Autodesk Inventor part; units mm, degrees
ref_plane "YZ Plane" through (0, 0, 0) normal (1, 0, 0) x (0, 1, 0)
ref_plane "XZ Plane" through (0, 0, 0) normal (0, 1, 0) x (-1, 0, 0)
ref_plane "XY Plane" through (0, 0, 0) normal (0, 0, 1) x (1, 0, 0)
ref_plane "Work Plane1" through (0, 0, 0) normal (0, 0, 1) x (1, 0, 0)
sketch "Sketch1" plane through (0, 0, 0) normal (0, 0, 1) x (1, 0, 0)
  circle A0 centre (6.5, 20.75) radius 1
  circle A1 centre (6.5, 4.75) radius 1
  circle A2 centre (22.5, 20.75) radius 1
  circle A3 centre (22.5, 4.75) radius 1
  line L0 (-13, -14.75) -> (43.896, -14.75)
  line L1 (43.896, -14.75) -> (43.896, 40.25)
  line L2 (43.896, 40.25) -> (-13, 40.25)
  line L3 (-13, 40.25) -> (-13, -14.75)
  circle A4 centre (22.5, 12.75) radius 1
  circle A5 centre (14.5, 20.75) radius 1
  circle A6 centre (14.5, 4.75) radius 1
  circle A7 centre (6.5, 12.75) radius 1
  point P0 (0, 0)
  point P1 (14.5, 12.75)
  dimension "d1" = 55
  dimension "d102" = 29.396
  dimension "d103" = 27.5
  dimension "d107" = 2
  dimension "d108" = 2
  dimension "d109" = 2
  dimension "d110" = 2
extrude "Extrusion3" add sketch "Sketch1" along normal blind 3
sketch "Sketch4" plane through (0, 0, 3) normal (0, 0, 1) x (1, 0, 0)
  line L0 (42, 40.25) -> (-13, 40.25) construction
  line L1 (14.5, 40.25) -> (14.5, 12.75) construction
  line L2 (-13, -14.75) -> (42, -14.75) construction
  line L3 (-13, 40.25) -> (-13, -14.75) construction
  line L4 (-13, 12.75) -> (14.5, 12.75) construction
  circle A0 centre (14.5, 30.75) radius 3.895
  circle A1 centre (1.7721, 25.4779) radius 3.895
  circle A2 centre (-3.5, 12.75) radius 3.895
  circle A3 centre (1.7721, 0.0221) radius 3.895
  circle A4 centre (14.5, -5.25) radius 3.895
  circle A5 centre (27.2279, 0.0221) radius 3.895
  circle A6 centre (32.5, 12.75) radius 3.895
  circle A7 centre (27.2279, 25.4779) radius 3.895
  arc A8 (4.6716, 35.75) -> (4.6716, 37.75) centre (7.5, 36.75) ccw
  line L5 (42, 40.25) -> (-13, 40.25)
  line L6 (7.5, 36.75) -> (-13, 36.75) construction
  line L7 (4.6716, 37.75) -> (-7.3284, 37.75)
  line L8 (4.6716, 35.75) -> (-7.3284, 35.75)
  line L9 (-7.3284, 37.75) -> (-7.3284, 40.25)
  line L10 (10.9716, 40.25) -> (-7.3284, 40.25)
  line L11 (-7.3284, 35.75) -> (-7.3284, 33.25)
  line L12 (-7.3284, 33.25) -> (10.9716, 33.25)
  line L13 (10.9716, 40.25) -> (10.9716, 33.25)
  arc A9 (24.3284, 37.75) -> (24.3284, 35.75) centre (21.5, 36.75) ccw
  line L14 (24.3284, 37.75) -> (36.3284, 37.75)
  line L15 (24.3284, 35.75) -> (36.3284, 35.75)
  line L16 (36.3284, 37.75) -> (36.3284, 40.25)
  line L17 (18.0284, 40.25) -> (36.3284, 40.25)
  line L18 (36.3284, 35.75) -> (36.3284, 33.25)
  line L19 (36.3284, 33.25) -> (18.0284, 33.25)
  line L20 (18.0284, 40.25) -> (18.0284, 33.25)
  arc A10 (-6.6716, -10.25) -> (-6.6716, -12.25) centre (-9.5, -11.25) ccw
  line L21 (-9.5, -11.25) -> (8.4531, -11.25) construction
  line L22 (-6.6716, -10.25) -> (5.3284, -10.25)
  line L23 (-6.6716, -12.25) -> (5.3284, -12.25)
  line L24 (5.3284, -12.25) -> (5.3284, -14.75)
  line L25 (5.3284, -10.25) -> (5.3284, -7.75)
  line L26 (5.3284, -7.75) -> (-13, -7.75)
  line L27 (-13, -14.75) -> (-13, -7.75)
  line L28 (-13, -14.75) -> (5.3284, -14.75)
  circle A11 centre (14.5, 12.75) radius 5
  point P0 (0, 0)
  dimension "d24" = 7.79
  dimension "d25" = 18
  dimension "d28" = 360
  dimension "d63" = 6
  dimension "d64" = 7
  dimension "d65" = 12
  dimension "d66" = 18.3
  dimension "d67" = 2.5
  dimension "d68" = 3.5
  dimension "d71" = 1
  dimension "d74" = 6
  dimension "d75" = 3.5
  dimension "d76" = 3.5
  dimension "d77" = 12
  dimension "d78" = 1
  dimension "d79" = 2.5
  dimension "d105" = 10
extrude "Extrusion2" cut sketch "Sketch4" against normal through all
hole "Hole4" at (7.5, 36.75, 3) at (21.5, 36.75, 3) at (-9.5, -11.25, 3) direction (0, 0, -1) diameter 2 end through all
fillet "Fillet3" radius 2 14 edges at (-7.3284, 35.75, 1.5) (-7.3284, 37.75, 1.5) (4.6716, 37.75, 1.5) (4.6716, 35.75, 1.5) (10.9716, 33.25, 1.5) (24.3284, 37.75, 1.5) (24.3284, 35.75, 1.5) (36.3284, 37.75, 1.5) (36.3284, 35.75, 1.5) (18.0284, 33.25, 1.5) (5.3284, -10.25, 1.5) (5.3284, -12.25, 1.5) (-6.6716, -10.25, 1.5) (-6.6716, -12.25, 1.5)
sketch "Sketch6" plane through (0, 0, 3) normal (0, 0, 1) x (1, 0, 0)
  line L0 (43.896, 40.25) -> (36.3284, 40.25)
  line L1 (43.896, 40.25) -> (40.796, 40.25)
  line L2 (40.796, 40.25) -> (40.796, 20.2)
  line L3 (40.796, 20.2) -> (43.896, 20.2)
  line L4 (43.896, 20.2) -> (43.896, 40.25)
  line L5 (43.896, -14.75) -> (43.896, 40.25) construction
  line L6 (43.896, 12.75) -> (-13, 12.75) construction
  line L7 (-13, 40.25) -> (-13, -7.75) construction
  line L8 (43.896, -14.75) -> (40.796, -14.75)
  line L9 (40.796, -7.75) -> (40.796, 5.3)
  line L10 (40.796, 5.3) -> (43.896, 5.3)
  line L11 (43.896, 5.3) -> (43.896, -14.75)
  line L12 (43.896, -14.75) -> (33.896, -14.75)
  line L13 (33.896, -14.75) -> (33.896, -7.75)
  line L14 (33.896, -7.75) -> (40.796, -7.75)
  line L15 (43.896, -7.75) -> (43.896, -14.75)
  point P0 (0, 0)
  dimension "d96" = 3.1
  dimension "d97" = 20.05
  dimension "d100" = 10
  dimension "d101" = 7
extrude "Extrusion4" cut sketch "Sketch6" against normal through all
fillet "Fillet4" radius 3 1 edges at (-13, 40.25, 1.5)
equation "\"d38\" = d24"
properties part number "Side"
The listing builds one solid part. Answer for the finished solid, in the listing's coordinates (mm). A direction names the side the tool comes from. Coordinates: 2 decimals unless noted, no trailing zeros. Write each loop counter-clockwise with the first axis right and the second up, starting at its lowest first coordinate (ties: lowest second). Pieces come first, ordered by that corner, then holes. Notation, with made-up numbers: (11.25, 42.25) -> (64.25, 42.25) arc R17 ccw to (64.25, 52.25) -> close; hole circle Ø3 at (75, 31.25). An arc over 180 degrees is marked (long way). Write each question's results on one line, items separated by ' | '. Start each with the question number.
1) A tool of negligible diameter and unlimited length cuts with its end or side. For faces 1 (the flat face through (-9, 40.25, 1)), 2 (the cylindrical face through (-6.727, 38.32, 1.479)), 3 (the flat face through (15, 19, 3)), 4 (the flat face through (28, 33.25, 2)), 5 (the cylindrical face through (-6.41, -12.47, 1.48)), from which of +Z, -Z, +X, -X, +Y, -Y can it reach the whole face along a straight path? Write none if from no direction.
2) For a pull along X with two mould halves and no side action, classify faces 6 (the flat face through (33.896, -11, 2)), 7 (the cylindrical face through (-12.1, 39.39, 1.52)), 8 (the cylindrical face through (23.337, 0.193, 1.521)), 9 (the flat face through (37, -7.75, 2)) as +X half, -X half, draft (parallel to the pull), parting line (faces both ways), or undercut.
3) A cutting plane is placed at C-C (y = 30.75). Determine the outline of the cut face in (x, z) (3 decimals), then the cut area to 3 significant figures.
4) Straight lines are drawn through the part: probe 1 along Y at (x, z) = (2, 2.2); probe 2 along Y at (x, z) = (-3.5, 0.75) (3 decimals); probe 3 along Y at (x, z) = (-9.5, 1.3). For each, find the intervals that lie inside material, in ascending order.
5) A cutting plane is placed at D-D (x = 32.5). Determine the outline of the cut face in (y, z) (3 decimals).
6) A cutting plane is placed at B-B (y = 12.75). Determine the outline of the cut face in (x, z) (3 decimals).
7) Flat-ended cylindrical pins translate along their axes: pin 1 Ø6 at (x, y) = (32.5, 12.75) entering from -Z; pin 2 Ø3 at (x, y) = (6.5, 4.75) entering from +Z; pin 3 Ø0.9 at (x, z) = (42, 1.5) entering from -Y; pin 4 Ø1 at (x, z) = (-6.5, 2.5) entering from -Y. Find the tip coordinate at first contact, or state that the pin passes through.
8) A cutting plane is placed at A-A (x = 14.5). Determine the outline of the cut face in (y, z) (3 decimals), then the cut area to 3 significant figures.
Values follow:
1) face 1: +Z, -Z, +X, -X, +Y | face 2: +Z, -Z, +Y | face 3: +Z, +X, -X, +Y, -Y | face 4: +Z, -Z | face 5: +Z, -Z, -Y
2) face 6: +X half | face 7: -X half | face 8: undercut | face 9: draft
3) outline: (-13, 0) -> (10.605, 0) -> (10.605, 3) -> (-13, 3) -> close; (18.395, 0) -> (40.796, 0) -> (40.796, 3) -> (18.395, 3) -> close | area: 138 mm²
4) probe 1: -12.25 to -10.25, -7.75 to -3.87, 3.91 to 21.59, 29.37 to 33.25, 35.75 to 37.75 | probe 2: -12.25 to -10.25, -7.75 to 8.855, 16.645 to 33.25, 35.75 to 37.75 | probe 3: -14.25 to -12.25, -10.25 to -8.25, -7.75 to 40.25
5) outline: (-14.75, 0) -> (8.855, 0) -> (8.855, 3) -> (-14.75, 3) -> close; (16.645, 0) -> (33.25, 0) -> (33.25, 3) -> (16.645, 3) -> close; (35.75, 0) -> (37.75, 0) -> (37.75, 3) -> (35.75, 3) -> close
6) outline: (-13, 0) -> (-7.395, 0) -> (-7.395, 3) -> (-13, 3) -> close; (0.395, 0) -> (5.5, 0) -> (5.5, 3) -> (0.395, 3) -> close; (7.5, 0) -> (9.5, 0) -> (9.5, 3) -> (7.5, 3) -> close; (19.5, 0) -> (21.5, 0) -> (21.5, 3) -> (19.5, 3) -> close; (23.5, 0) -> (28.605, 0) -> (28.605, 3) -> (23.5, 3) -> close; (36.395, 0) -> (43.896, 0) -> (43.896, 3) -> (36.395, 3) -> close
7) pin 1: through | pin 2: z = 3 | pin 3: y = 5.3 | pin 4: y = -12.93
8) outline: (-14.75, 0) -> (-9.145, 0) -> (-9.145, 3) -> (-14.75, 3) -> close; (-1.355, 0) -> (3.75, 0) -> (3.75, 3) -> (-1.355, 3) -> close; (5.75, 0) -> (7.75, 0) -> (7.75, 3) -> (5.75, 3) -> close; (17.75, 0) -> (19.75, 0) -> (19.75, 3) -> (17.75, 3) -> close; (21.75, 0) -> (26.855, 0) -> (26.855, 3) -> (21.75, 3) -> close; (34.645, 0) -> (40.25, 0) -> (40.25, 3) -> (34.645, 3) -> close | area: 76.3 mm²
